from build123d import *

# Parameters (mm, degrees)
BOSS_EXTRUDE1_DEPTH = 150
SKETCH2_R           = 2
CUT_EXTRUDE1_DEPTH  = 10


with BuildPart() as part:
    # Sketch1 → Boss-Extrude1 (new body)
    with BuildSketch(Plane.XY):
        Polygon((0, 0), (0, 20), (20, 20), (20, 18.8), (1.2, 18.8), (1.2, 0), align=None)
    extrude(amount=BOSS_EXTRUDE1_DEPTH)

    # Sketch2 → Cut-Extrude1 (cut)
    with BuildSketch(Plane(origin=(0, 20, 0), x_dir=(1, 0, 0), z_dir=(0, 1, 0))):
        with Locations(Location((10, -75, 0), (0, 0, 270))):
            Circle(SKETCH2_R)
        with Locations(Location((10, -10, 0), (0, 0, 270))):
            Circle(SKETCH2_R)
        with Locations(Location((10, -140, 0), (0, 0, 270))):
            Circle(SKETCH2_R)
    extrude(amount=-CUT_EXTRUDE1_DEPTH, mode=Mode.SUBTRACT)


solid = part.part
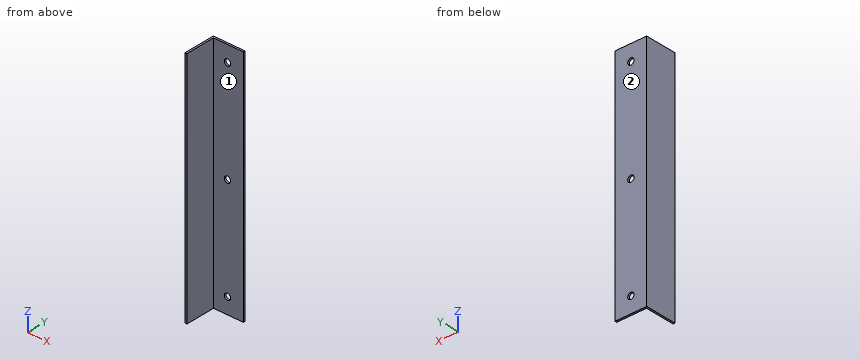
Design review of the part built by this model. Coordinates are the model's own, in mm. Face numbers are marked on the shaded views. A direction names the side the tool comes from. Coordinates: 2 decimals unless noted, no trailing zeros. Loops run counter-clockwise (first coordinate to the right, second up) from the corner with the lowest first, then second, coordinate; pieces in that order, holes last. Notation, with made-up numbers: M 43,12 L 75,12 A12 cw 75,16 Z; hole C 76,61.25 d4. An arc over 180 degrees is marked long. Use one line per item in the form item = value.
(1) For line 1 along X through (y, z) = (19.3, 10); line 2 along X through (y, z) = (17.75, 134); line 3 along Y through (x, z) = (19, 112.5), list the stretches that pass through material, from the lowest coordinate up. Write a range as from..to.
Return value:
line_1 = 0..8, 12..20
line_2 = 0..1.2
line_3 = 18.8..20
(2) Clearance check with flat-ended pins moving along their axes: P1, Ø6, axis at x = 3.5, z = 61.5, coming from the -Y side; P2, Ø5.5, axis at y = 13, z = 59.5, coming from the +X side; P3, Ø8, axis at x = 12.5, z = 29, coming from the -Y side. State where each tip first meets the part, or that it passes through.
Return value:
P1 = 0
P2 = 1.2
P3 = 18.8
(3) Consider section A-A (x = 10). Write out the cut boundary in (y, z), and give its area (3 significant figures).
Return value:
outline = M 18.8,0 L 20,0 L 20,8 L 18.8,8 Z; M 18.8,12 L 20,12 L 20,73 L 18.8,73 Z; M 18.8,77 L 20,77 L 20,138 L 18.8,138 Z; M 18.8,142 L 20,142 L 20,150 L 18.8,150 Z
area = 166 mm2
(4) Consider section C-C (z = 80). Write out the cut boundary in (x, y).
Return value:
outline = M 0,0 L 1.2,0 L 1.2,18.8 L 20,18.8 L 20,20 L 0,20 Z
(5) For the marked faces 1 and 2, list the 3-axis set-ups (+Z, -Z, +X, -X, +Y, -Y) from which the entire face can be reached by the end or side of a thin tool; tool diameter is ignored.
Return value:
face_1 = +Z, -Z, +X, -Y
face_2 = +Z, -Z, +X, -X, +Y
(6) Consider section D-D (y = 13.5). Write out the cut boundary in (x, z), and give its area (3 significant figures).
Return value:
outline = M 0,0 L 1.2,0 L 1.2,150 L 0,150 Z
area = 180 mm2
(7) Consider section B-B (z = 10). Write out the cut boundary in (x, y), and give its area (3 significant figures).
Return value:
outline = M 0,0 L 1.2,0 L 1.2,18.8 L 8,18.8 L 8,20 L 0,20 Z; M 12,18.8 L 20,18.8 L 20,20 L 12,20 Z
area = 41.8 mm2
